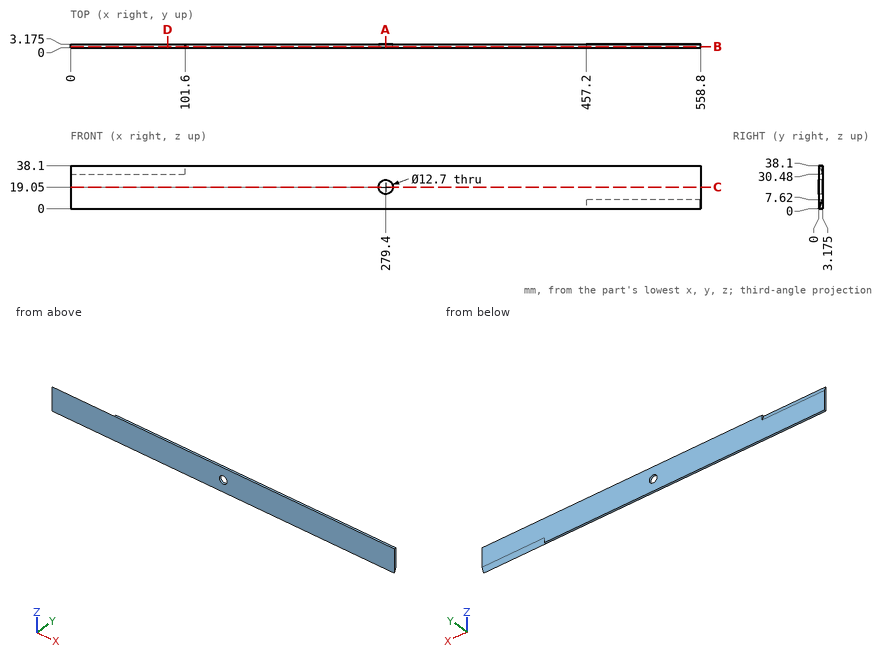
Geometry: see drawing. Coordinates: mm, zero at the bounding-box minimum. Coordinates: 2 decimals unless noted, no trailing zeros. Loops run counter-clockwise (first coordinate to the right, second up) from the corner with the lowest first, then second, coordinate; pieces in that order, holes last. Notation, with made-up numbers: M -36.5,63 L -30.5,63 A35 cw -30.5,97 Z; hole C 74.5,73.25 d1. An arc over 180 degrees is marked long. Put each result on its own line as item: value. Start each with the question number.
1) Cut plane B-B on y = 0.75. Return the cut outline in (x, z).
2) Ray query, L1, parallel to Z at x = 279.4, y = 2.25; L2, parallel to X at y = 1.1, z = 19.05; L3, parallel to X at y = 2.05, z = 22.5. Return the intervals inside material, ascending. Write a range as from..to.
3) Cut plane A-A on x = 279.4. Return the cut outline in (y, z) (3 decimals).
4) Cut plane D-D on x = 86. Return the cut outline in (y, z) (3 decimals), then the cut area to 3 significant figures.
5) Cut plane C-C on z = 19.05. Return the cut outline in (x, y) (3 decimals), then the cut area to 3 significant figures.
The answers:
1. outline: M 0,0 L 457.2,0 L 457.2,1.8 L 558.8,1.8 L 558.8,38.1 L 101.6,38.1 L 101.6,36.3 L 0,36.3 Z; hole C 279.4,19.05 d12.7
2. L1: z = 0..12.7, 25.4..38.1
2. L2: x = 0..273.05, 285.75..558.8
2. L3: x = 0..274.07, 284.73..558.8
3. outline: M 0,0 L 3.175,0 L 3.175,12.7 L 0,12.7 Z; M 0,25.4 L 3.175,25.4 L 3.175,38.1 L 0,38.1 Z
4. outline: M 0,0 L 3.175,0 L 3.175,30.48 L 0,38.1 Z
4. area: 109 mm²
5. outline: M 0,0 L 273.05,0 L 273.05,3.175 L 0,3.175 Z; M 285.75,0 L 558.8,0 L 558.8,3.175 L 285.75,3.175 Z
5. area: 1,730 mm²
